from build123d import *

# Parameters (mm, degrees)
F0_W     = 30
F0_H     = 6
F1_DEPTH = 150
F2_W     = 3
F2_H     = 50
F3_DEPTH = 30
F4_W     = 5
F4_H     = 5
F5_DEPTH = 3


with BuildPart() as f1:
    # F0 (on Top) → F1 (new body)
    with BuildSketch(Plane.XY):
        Rectangle(F0_W, F0_H)
    extrude(amount=F1_DEPTH)

    # F2 (on face) → F3 (cut, through all)
    with BuildSketch(Plane.YZ.offset(15)):
        with Locations((1.5, 125)):
            Rectangle(F2_W, F2_H)
        with Locations((1.5, 25)):
            Rectangle(F2_W, F2_H)
    extrude(amount=-F3_DEPTH, mode=Mode.SUBTRACT)

    # F4 (on face) → F5 (cut, through all)
    with BuildSketch(Plane(origin=(0, 0, 0), x_dir=(-1, 0, 0), z_dir=(0, 1, 0))):
        with Locations((7.5, 12.5)):
            Rectangle(F4_W, F4_H)
        with Locations((-7.5, 12.5)):
            Rectangle(F4_W, F4_H)
        with Locations((-7.5, 42.5)):
            Rectangle(F4_W, F4_H)
        with Locations((7.5, 42.5)):
            Rectangle(F4_W, F4_H)
        with Locations((7.5, 107.5)):
            Rectangle(F4_W, F4_H)
        with Locations((-7.5, 107.5)):
            Rectangle(F4_W, F4_H)
        with Locations((-7.5, 137.5)):
            Rectangle(F4_W, F4_H)
        with Locations((7.5, 137.5)):
            Rectangle(F4_W, F4_H)
    extrude(amount=-F5_DEPTH, mode=Mode.SUBTRACT)


solid = f1.part
Input: part model. Units: mm. Frame: model coordinates. A direction names the side the tool comes from. Give positions to 0.01 mm unless a question says otherwise; leave off trailing zeros. Loops run counter-clockwise (first coordinate to the right, second up) from the corner with the lowest first, then second, coordinate; pieces in that order, holes last. Notation, with made-up numbers: (37, 63.5) - (72, 63.5) arc R30 cw to (72, 97.5) - close; hole circle Ø2 at (30, -23). An arc over 180 degrees is marked (long way). Use CSV: the item, a comma, the result in double quotes. Start each with the question number.
Item 1: Contact query for flat-ended pins moving along their axis: P1, Ø0.9, axis at x = 6.5, y = -1, coming from the -Z side; P2, Ø9, axis at x = 1.5, z = 128, coming from the +Y side. Output: stop coordinate, or through.
Item 2: Section C-C on z = 18. Return loops of the section in (x, y), then the cut area to 3 significant figures.
Item 3: Section A-A on x = 6.25. Return loops of the section in (y, z).
Item 4: Mould query, pull axis Z, two halves, no side actions, for faces 4 (the flat face through (0, 1, 50)), 5 (the flat face through (8, -1, 105)), 6 (the flat face through (15, -1, 74)). Classes: pulls with the +Z half, pulls with the -Z half, needs draft (parallel to the pull), parting line crosses it, or undercut.
Item 5: Section B-B on y = 1.35. Return loops of the section in (x, z), then the cut area to 3 significant figures.
Item 6: Reachability of faces 1 (the flat face through (0, -1, 0)), 2 (the flat face through (-5, -1, 42)), 3 (the flat face through (0, 1, 100)) from +Z, -Z, +X, -X, +Y, -Y: full face, straight path, thin tool, end or side. Return the list, or none.
Item 7: Line query: line 1 (Z direction, x = -9.5, y = -1.45); line 2 (X direction, y = -0.4, z = 12); line 3 (Y direction, x = -0.25, z = 14). Output: solid intervals per line, ascending.
Ans:
1,P1,"stops at z = 0"
1,P2,"stops at y = 0"
2,outline,"(-15, -3) - (15, -3) - (15, 0) - (-15, 0) - close"
2,area,"90.0 mm2"
3,outline,"(-3, 0) - (0, 0) - (0, 10) - (-3, 10) - close; (-3, 15) - (0, 15) - (0, 40) - (-3, 40) - close; (-3, 45) - (0, 45) - (0, 50) - (3, 50) - (3, 100) - (0, 100) - (0, 105) - (-3, 105) - close; (-3, 110) - (0, 110) - (0, 135) - (-3, 135) - close; (-3, 140) - (0, 140) - (0, 150) - (-3, 150) - close"
4,face 4,"pulls with the -Z half"
4,face 5,"undercut"
4,face 6,"needs draft"
5,outline,"(-15, 50) - (15, 50) - (15, 100) - (-15, 100) - close"
5,area,"1,500 mm2"
6,face 1,"-Z, +X, -X, +Y, -Y"
6,face 2,"+Y, -Y"
6,face 3,"+Z, +X, -X, +Y"
7,line 1,"z = 0 to 10, 15 to 40, 45 to 105, 110 to 135, 140 to 150"
7,line 2,"x = -15 to -10, -5 to 5, 10 to 15"
7,line 3,"y = -3 to 0"
